Answer from the drawing. Dimensions are ordinates in mm from the lowest x, y and z of the part. Give positions to 0.01 mm unless a question says otherwise; leave off trailing zeros. Order: outer loops, then holes, each group sorted by start corner. A loop starts at its lowest first (then second) coordinate and runs counter-clockwise, first axis right, second up. Notation, with made-up numbers: M -24,27 L 9,27 A20 ccw 9,59 Z; hole C 54,50 d8. An arc over 180 degrees is marked long. One line per item, written item: value.
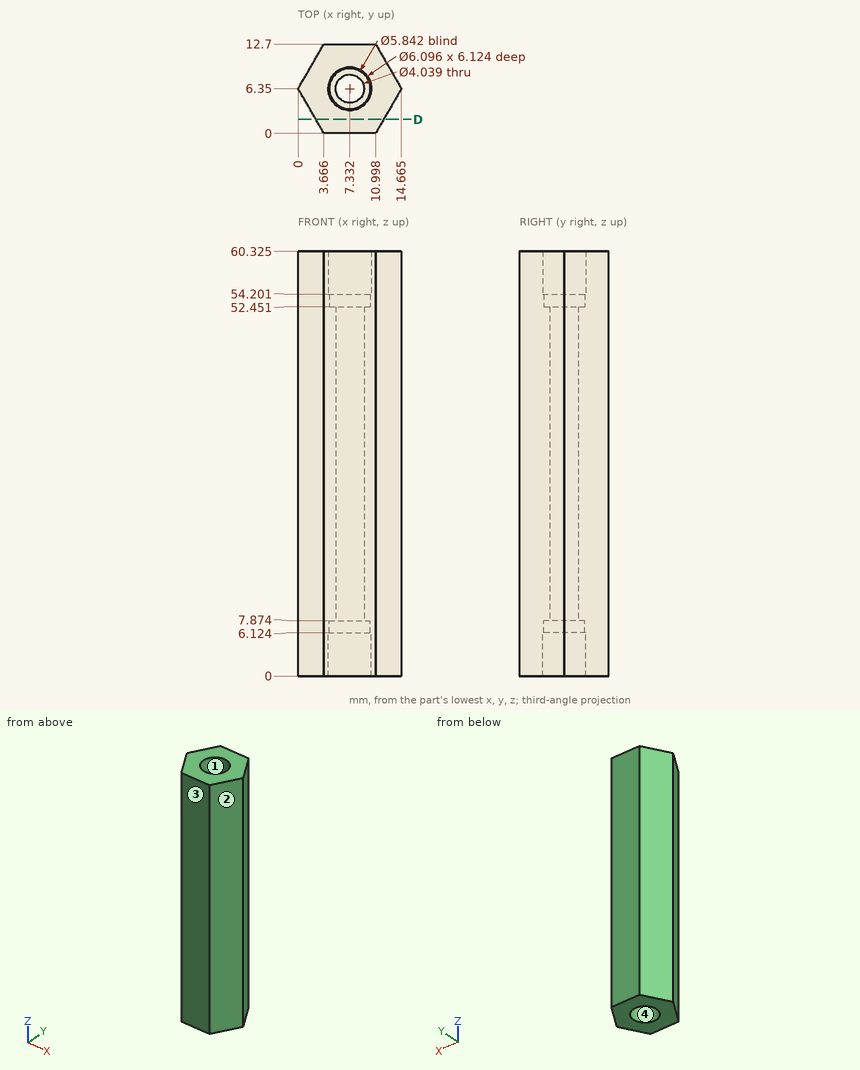
(1) Section D-D, the plane y = 2 is taken. Give the vertices of the cut face in (x, z) (1 decimal).
Findings:
outline: M 2.5,0 L 12.2,0 L 12.2,60.3 L 2.5,60.3 Z
(2) Given P1, Ø5, axis at y = 11, z = 25.5, coming from the +X side; P2, Ø5, axis at x = 7.33, y = 6.35, coming from the -Z side; P3, Ø2, axis at x = 2, z = 37.5, coming from the -Y side (1 decimal), each flat-ended and moving along its own axis, determine where each tip first touches the part or whether it passes through.
Findings:
P1: stops at x = 13.42
P2: stops at z = 7.87
P3: stops at y = 1.2
(3) Determine the mould class of the marked faces 1, 2, 3 and 4 for opening direction X: pulls with the +X half, pulls with the -X half, needs draft (parallel to the pull), parting line crosses it, or undercut.
Findings:
face 1: undercut
face 2: pulls with the +X half
face 3: needs draft
face 4: undercut
(4) Find the intervals of material crossed by probe 1 along Z at (x, y) = (5.25, 8.5); probe 2 along X at (y, z) = (5.75, 23) (1 decimal); probe 3 along Y at (x, z) = (7, 44), in increasing order. Write a range as from..to.
Findings:
probe 1: z = 6.12..54.2
probe 2: x = 0.3..5.4, 9.3..14.3
probe 3: y = 0..4.36, 8.34..12.7
